```python
from build123d import *

# Parameters (mm, degrees)
SKETCH1_R           = 7
BOSS_EXTRUDE1_DEPTH = 46.228
SKETCH2_R           = 9
BOSS_EXTRUDE2_DEPTH = 5
SKETCH3_W           = 14
SKETCH3_H           = 10
BOSS_EXTRUDE3_DEPTH = 9.5
SKETCH4_OUTSIDE_W   = 33.17
SKETCH4_OUTSIDE_H   = 33.17
SKETCH4_OUTSIDE_W_2 = 11
SKETCH4_OUTSIDE_H_2 = 11
CUT_EXTRUDE1_DEPTH  = 29.464
SKETCH5_R           = 3.81
CUT_EXTRUDE2_DEPTH  = 64.080424729


with BuildPart() as part:
    # Sketch1 → Boss-Extrude1 (new body)
    with BuildSketch(Plane(origin=(0, 0, 0), x_dir=(1, 0, 0), z_dir=(0, 1, 0))):
        with Locations(Location((0, 0, 0), (0, 0, 270))):
            Circle(SKETCH1_R)
    extrude(amount=BOSS_EXTRUDE1_DEPTH)

    # Sketch2 → Boss-Extrude2 (add, symmetric)
    with BuildSketch(Plane(origin=(0, 46.228, 0), x_dir=(1, 0, 0), z_dir=(0, 1, 0))):
        with Locations(Location((0, 0, 0), (0, 0, 270))):
            Circle(SKETCH2_R)
    extrude(amount=BOSS_EXTRUDE2_DEPTH, both=True)

    # Sketch3 → Boss-Extrude3 (add)
    with BuildSketch(Plane(origin=(0, 51.228, 0), x_dir=(1, 0, 0), z_dir=(0, 1, 0))):
        Rectangle(SKETCH3_W, SKETCH3_H)
    extrude(amount=BOSS_EXTRUDE3_DEPTH)

    # Sketch4 outside → Cut-Extrude1 (cut)
    with BuildSketch(Plane(origin=(0, 0, 0), x_dir=(1, 0, 0), z_dir=(0, 1, 0))):
        Rectangle(SKETCH4_OUTSIDE_W, SKETCH4_OUTSIDE_H)
        Rectangle(SKETCH4_OUTSIDE_W_2, SKETCH4_OUTSIDE_H_2, mode=Mode.SUBTRACT)
    extrude(amount=CUT_EXTRUDE1_DEPTH, mode=Mode.SUBTRACT)

    # Sketch5 → Cut-Extrude2 (cut, through all)
    with BuildSketch(Plane(origin=(0, 0, -5.5), x_dir=(-1, 0, 0), z_dir=(0, 0, -1))):
        with Locations((0, 11.43)):
            Circle(SKETCH5_R)
    extrude(amount=-CUT_EXTRUDE2_DEPTH, mode=Mode.SUBTRACT)


solid = part.part
```
Input: part model. Units: mm. Frame: model coordinates. A direction names the side the tool comes from. Coordinates: 2 decimals unless noted, no trailing zeros. Order: outer loops, then holes, each group sorted by start corner. A loop starts at its lowest first (then second) coordinate and runs counter-clockwise, first axis right, second up. Notation, with made-up numbers: (-25.5, -8) - (10.5, -8) arc R27 cw to (10.5, 29) - close; hole circle Ø6 at (-31, 57.25). An arc over 180 degrees is marked (long way). Return JSON: item names as keys, results as strings.
Q1. Ray query, probe 1 along Y at (x, z) = (0, 1.75); probe 2 along Y at (x, z) = (-2.25, -7); probe 3 along X at (y, z) = (14.5, 4). Return the intervals inside material, ascending.
The answers:
{"probe 1": "y = 0 to 7.62, 15.24 to 60.73", "probe 2": "y = 41.23 to 51.23", "probe 3": "x = -5.5 to -2.26, 2.26 to 5.5"}
Q2. Cut plane D-D (y = 52). Return loops of the section in (x, z), then the cut area to 3 significant figures.
The answers:
{"outline": "(-7, -5) - (7, -5) - (7, 5) - (-7, 5) - close", "area": "140 mm2"}
Q3. Cut plane B-B (x = 0). Return loops of the section in (y, z), then the cut area to 3 significant figures.
The answers:
{"outline": "(0, -5.5) - (7.62, -5.5) - (7.62, 5.5) - (0, 5.5) - close; (15.24, -5.5) - (29.46, -5.5) - (29.46, -7) - (41.23, -7) - (41.23, -9) - (51.23, -9) - (51.23, -5) - (60.73, -5) - (60.73, 5) - (51.23, 5) - (51.23, 9) - (41.23, 9) - (41.23, 7) - (29.46, 7) - (29.46, 5.5) - (15.24, 5.5) - close", "area": "680 mm2"}
Q4. Cut plane C-C (z = 0). Return loops of the section in (x, y).
The answers:
{"outline": "(-9, 41.23) - (-7, 41.23) - (-7, 29.46) - (-5.5, 29.46) - (-5.5, 0) - (5.5, 0) - (5.5, 29.46) - (7, 29.46) - (7, 41.23) - (9, 41.23) - (9, 51.23) - (7, 51.23) - (7, 60.73) - (-7, 60.73) - (-7, 51.23) - (-9, 51.23) - close; hole circle Ø7.62 at (0, 11.43)"}
Q5. Cut plane A-A (y = 11.43). Return loops of the section in (x, z), then the cut area to 3 significant figures.
The answers:
{"outline": "(-5.5, -4.33) arc R7 ccw to (-4.33, -5.5) - (-3.81, -5.5) - (-3.81, 5.5) - (-4.33, 5.5) arc R7 ccw to (-5.5, 4.33) - close; (3.81, -5.5) - (4.33, -5.5) arc R7 ccw to (5.5, -4.33) - (5.5, 4.33) arc R7 ccw to (4.33, 5.5) - (3.81, 5.5) - close", "area": "34.7 mm2"}
Q6. First-contact query: pin 1 (1.5 mm diameter, centred on x = 6, y = 23.5, fed in from +Z); pin 2 (4.5 mm diameter, centred on x = 0, y = 11.43, fed in from +Z); pin 3 (7.5 mm diameter, centred on y = 58, z = 1, fed in from -X); pin 4 (6 mm diameter, centred on x = -4, y = 19, fed in from -Z). Flat tips, straight axial feed; report the tip coordinate or a pass-through.
The answers:
{"pin 1": "stops at z = 4.63", "pin 2": "passes through", "pin 3": "stops at x = -7", "pin 4": "stops at z = -5.5"}
Q7. Draft query along Y for faces 6 (the flat face through (0, 60.728, 0)), 7 (the flat face through (0, 29.464, -6)), 8 (the cylindrical face through (0.83, 7.71, -0.08)), 9 (the cylindrical face through (2.703, 46.298, 8.584)). Return one class per face: +Y half, -Y half, draft (parallel to the pull), parting line (faces both ways), or undercut.
The answers:
{"face 6": "+Y half", "face 7": "-Y half", "face 8": "undercut", "face 9": "draft"}
Q8. Access query for faces 1 (the flat face through (0, 18, -5.5)), 2 (the flat face through (0, 56, 5)), 3 (the flat face through (-6, 29.464, 0)), 4 (the flat face through (7, 56, 0)), 5 (the flat face through (-7, 56, 0)). Directions: +Z, -Z, +X, -X, +Y, -Y. A direction counts if a zero-diameter tool reaches every point of the face in a straight line with its end or side. Return the directions, or none.
The answers:
{"face 1": "-Z, +X, -X, -Y", "face 2": "+Z, +X, -X, +Y", "face 3": "+Z, -Z, -X, -Y", "face 4": "+Z, -Z, +X, +Y", "face 5": "+Z, -Z, -X, +Y"}
